Check sheet for the modelled part. Datum: model origin and axes. Units: mm. Round coordinates to 2 decimals unless told otherwise and drop trailing zeros. Write each loop counter-clockwise with the first axis right and the second up, starting at its lowest first coordinate (ties: lowest second). Pieces come first, ordered by that corner, then holes.
Item 1: Section check C-C, the plane y = 19.75. Record the cut outline in (x, z).
Item 2: Material ranges on line 1 along Y through (x, z) = (-40.5, 3.6); line 2 along X through (y, z) = (19.75, 1.7); line 3 along Y through (x, z) = (-39.75, 2.9), recorded low to high.
Item 3: Section check D-D, the plane x = -43. Record the cut outline in (y, z).
Item 4: Section check A-A, the plane x = -39. Record the cut outline in (y, z), plus the area to 3 significant figures.
Item 5: Release check for a two-part mould opening along Y. For faces 1 (the cylindrical face through (-41.59, 19.32, 2.35)), 2 (the flat face through (-38.8, 17.8, 4.762)), 3 (the flat face through (-40.686, 12.775, 2.348)), 4 (the flat face through (-36.75, 24.25, 2.35)) record: pulls with the +Y half, pulls with the -Y half, needs draft (parallel to the pull), parting line crosses it, or undercut.
Item 6: Section check B-B, the plane z = 1.25. Record the cut outline in (x, y) (1 decimal), plus the area to 3 significant figures.
Item 7: Depth check by flat-ended pin: pin 1 (1.5 mm diameter, centred on x = -39.5, z = 3, fed in from -Y); pin 2 (1.5 mm diameter, centred on x = -35.5, y = 24, fed in from -Z); pin 3 (2 mm diameter, centred on x = -45, z = 2.5, fed in from +Y); pin 4 (2 mm diameter, centred on x = -37.5, z = 2, fed in from +Y). Enter the tip coordinate at first touch or a pass-through.
from build123d import *

# Parameters (mm, degrees)
F2_DEPTH = 4.7625
F3_R     = 1.5875
F4_DEPTH = 18.034


with BuildPart() as f2:
    # F0 (on Top) → F2 (new body)
    with BuildSketch(Plane.XY):
        Polygon((-37.663776, 12.472862), (-33.481061, 16.761916), (-34.2265, 22.706276), (-39.33876, 25.829716), (-44.968207, 23.780223), (-46.875751, 18.101107), (-43.624973, 13.068858), align=None)
    extrude(amount=F2_DEPTH)

    # F3 (on Top) → F4 (cut)
    with BuildSketch(Plane.XY):
        with Locations((-40.003754, 19.251533)):
            Circle(F3_R)
    extrude(amount=F4_DEPTH, mode=Mode.SUBTRACT)


solid = f2.part
Values found:
1. outline: (-46.32, 0) - (-41.51, 0) - (-41.51, 4.76) - (-46.32, 4.76) - close; (-38.5, 0) - (-33.86, 0) - (-33.86, 4.76) - (-38.5, 4.76) - close
2. line 1: y = 12.76 to 17.74, 20.76 to 25.41
2. line 2: x = -46.32 to -41.51, -38.5 to -33.86
2. line 3: y = 12.68 to 17.68, 20.82 to 25.68
3. outline: (13.01, 0) - (24.5, 0) - (24.5, 4.76) - (13.01, 4.76) - close
4. outline: (12.61, 0) - (18.02, 0) - (18.02, 4.76) - (12.61, 4.76) - close; (20.48, 0) - (25.62, 0) - (25.62, 4.76) - (20.48, 4.76) - close
4. area: 50.3 mm2
5. face 1: undercut
5. face 2: needs draft
5. face 3: pulls with the -Y half
5. face 4: pulls with the +Y half
6. outline: (-46.9, 18.1) - (-43.6, 13.1) - (-37.7, 12.5) - (-33.5, 16.8) - (-34.2, 22.7) - (-39.3, 25.8) - (-45, 23.8) - close; hole circle Ø3.2 at (-40, 19.3)
6. area: 123 mm2
7. pin 1: stops at y = 12.58
7. pin 2: stops at z = 0
7. pin 3: stops at y = 24.13
7. pin 4: stops at y = 25.32
